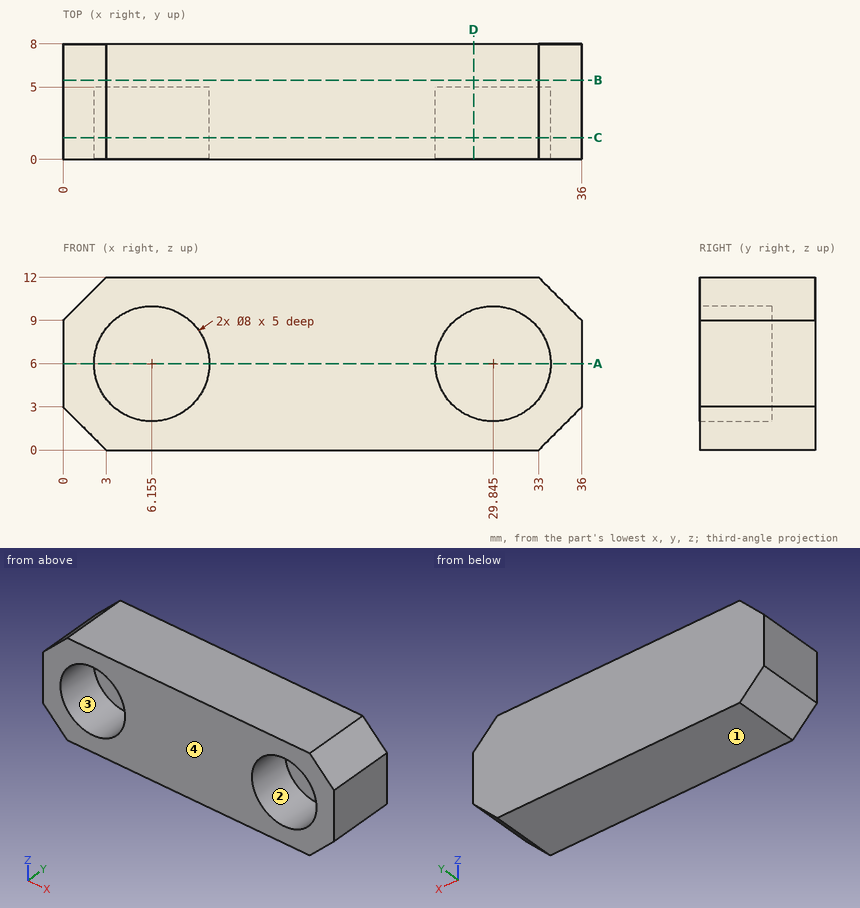
Part print with two shaded views. Sizes in mm from the minimum x, y, z corner. Round coordinates to 2 decimals unless told otherwise and drop trailing zeros. Loops run counter-clockwise (first coordinate to the right, second up) from the corner with the lowest first, then second, coordinate; pieces in that order, holes last.
1. Slice it at A-A (z = 6). Give the cut face in (x, y) (3 decimals).
Solutions:
outline: (0, 0) - (2.155, 0) - (2.155, 5) - (10.155, 5) - (10.155, 0) - (25.845, 0) - (25.845, 5) - (33.845, 5) - (33.845, 0) - (36, 0) - (36, 8) - (0, 8) - close
2. Slice it at B-B (y = 5.5). Give the cut face in (x, z).
Solutions:
outline: (0, 3) - (3, 0) - (33, 0) - (36, 3) - (36, 9) - (33, 12) - (3, 12) - (0, 9) - close
3. Slice it at C-C (y = 1.5). Give the cut face in (x, z) (3 decimals).
Solutions:
outline: (0, 3) - (3, 0) - (33, 0) - (36, 3) - (36, 9) - (33, 12) - (3, 12) - (0, 9) - close; hole circle Ø8 at (6.155, 6); hole circle Ø8 at (29.845, 6)
4. Slice it at D-D (x = 28.5). Give the cut face in (y, z).
Solutions:
outline: (0, 0) - (8, 0) - (8, 12) - (0, 12) - (0, 9.77) - (5, 9.77) - (5, 2.23) - (0, 2.23) - close
5. Drill centre lines: line 1 along X through (y, z) = (2.05, 6) (3 decimals); line 2 along X through (y, z) = (4.75, 6.5); line 3 along Y through (x, z) = (33.5, 7.25). Where is each one in solid material? Low to high.
Solutions:
line 1: x = 0 to 2.155, 10.155 to 25.845, 33.845 to 36
line 2: x = 0 to 2.19, 10.12 to 25.88, 33.81 to 36
line 3: y = 5 to 8
6. Two-plate mould, pull along Z, no slides. Class the marked faces 1, 2, 3 and 4: pulls with the +Z half, pulls with the -Z half, needs draft (parallel to the pull), parting line crosses it, or undercut.
Solutions:
face 1: pulls with the -Z half
face 2: undercut
face 3: undercut
face 4: needs draft
7. Flat gauge pin, fed straight in: pin 1 (5 mm diameter, centred on x = 29.845, z = 6, fed in from -Y). Where does the tip first touch, or does it go through?
Solutions:
pin 1: stops at y = 5
